Part model, mm, in its own coordinate system. A direction names the side the tool comes from. Give positions to 0.01 mm unless a question says otherwise; leave off trailing zeros. Write each loop counter-clockwise with the first axis right and the second up, starting at its lowest first coordinate (ties: lowest second). Pieces come first, ordered by that corner, then holes. Notation, with made-up numbers: (56, 84) - (110, 84) arc R12 ccw to (110, 105) - close; hole circle Ø2 at (18.25, 50). An arc over 180 degrees is marked (long way). Answer in a Markdown table with one row per item. Add a question column.
1. Pull direction Y, two halves, no side cores. Call faces 5 (the cylindrical face through (3.22, 1.01, 3.03)), 6 (the conical face through (1.35, 3.27, 5.16)), 7 (the flat face through (6.7, -0.1, 1.2)), 8 (the flat face through (0, 8, 3)): released by +Y, released by -Y, zero draft, split by the parting line, or undercut.
2. Band-saw the part on D-D on x = -7. Write the cut outline in (y, z).
3. Band-saw the part on B-B on z = 3. Write the cut outline in (x, y) (3 decimals), plus the area to 3 significant figures.
4. Band-saw the part on A-A on y = 0. Write the cut outline in (x, z) (3 decimals).
5. Probe line 1 along X through (y, z) = (0, 3.55) (3 decimals); line 2 along Y through (x, z) = (-1.5, 1.5). List the from-to ranges inside material, lowest first.
6. Drop flat-ended pins along their axis: pin 1 Ø1.7 at (x, y) = (-6, 2) entering from +Z; pin 2 Ø1.4 at (y, z) = (-0.5, 5) entering from -X; pin 3 Ø1 at (y, z) = (3, 5.5) entering from +X. Give the stop position or say it passes through.
7. Band-saw the part on C-C on y = 5.25. Write the cut outline in (x, z), plus the area to 3 significant figures.
8. Which spindle directions (+Z, -Z, +X, -X, +Y, -Y) get a long thin tool onto all of the face, cutting with end or side? Do faces 1 (the flat face through (4, 0, 5)), 2 (the flat face through (-6.8, -0.1, 1.3)), 3 (the flat face through (-6, 0, 4.1)), 4 (the flat face through (-0.493, 5.868, 5.706)). Say none if no direction does.
```python
from build123d import *

# Parameters (mm, degrees)
PAD_DEPTH   = 8
SKETCH001_R = 3.375
HOLE_DEPTH  = 6.001


with BuildPart() as part:
    # Sketch → Pad (new body, symmetric)
    with BuildSketch(Plane.XZ):
        with BuildLine():
            Line((-1, 6), (-3.7, 6))
            ThreePointArc((-3.7, 6), (-3.912132, 5.912132), (-4, 5.7))
            Line((-4, 5.7), (-4, 4.4))
            ThreePointArc((-4.3, 4.1), (-4.087868, 4.187868), (-4, 4.4))
            Line((-4.3, 4.1), (-7.7, 4.1))
            ThreePointArc((-7.7, 4.1), (-7.912132, 4.012132), (-8, 3.8))
            Line((-8, 3.8), (-8, 2.624264))
            ThreePointArc((-8, 2.624264), (-7.977164, 2.509459), (-7.912132, 2.412132))
            Line((-7.912132, 2.412132), (-5.587868, 0.087868))
            ThreePointArc((-5.587868, 0.087868), (-5.490541, 0.022836), (-5.375736, 0))
            Line((-5.375736, 0), (5.375736, 0))
            ThreePointArc((5.375736, 0), (5.490541, 0.022836), (5.587868, 0.087868))
            Line((5.587868, 0.087868), (7.912132, 2.412132))
            ThreePointArc((7.912132, 2.412132), (7.977164, 2.509459), (8, 2.624264))
            Line((8, 2.624264), (8, 3.8))
            ThreePointArc((8, 3.8), (7.912132, 4.012132), (7.7, 4.1))
            Line((7.7, 4.1), (4.3, 4.1))
            ThreePointArc((4, 4.4), (4.087868, 4.187868), (4.3, 4.1))
            Line((4, 4.4), (4, 5.7))
            ThreePointArc((4, 5.7), (3.912132, 5.912132), (3.7, 6))
            Line((3.7, 6), (1, 6))
            Line((1, 6), (0, 5.42))
            Line((0, 5.42), (-1, 6))
        make_face()
    extrude(amount=PAD_DEPTH, both=True)

    # Sketch001 → Hole (cut, through all)
    with BuildSketch(Plane.XY.offset(6)):
        Circle(SKETCH001_R)
    extrude(amount=-HOLE_DEPTH, mode=Mode.SUBTRACT)

    # Sketch002 → Groove (revolve, cut)
    with BuildSketch(Plane.YZ):
        Polygon((3.375, 6), (4.375, 6), (3.375, 5), align=None)
        Polygon((3.375, 0), (3.375, 1), (4.375, 0), align=None)
    revolve(axis=Axis((0, 0, 0), (0, 0, 1)), mode=Mode.SUBTRACT)


solid = part.part
```
Values:
| question | item | result |
|---|---|---|
| 1 | face 5 | undercut |
| 1 | face 6 | undercut |
| 1 | face 7 | zero draft |
| 1 | face 8 | released by +Y |
| 2 | outline | (-8, 1.5) - (8, 1.5) - (8, 4.1) - (-8, 4.1) - close |
| 3 | outline | (-8, -8) - (8, -8) - (8, 8) - (-8, 8) - close; hole circle Ø6.75 at (0, 0) |
| 3 | area | 220 mm² |
| 4 | outline | (-8, 2.624) arc R0.3 ccw to (-7.912, 2.412) - (-5.588, 0.088) arc R0.3 ccw to (-5.376, 0) - (-4.375, 0) - (-3.375, 1) - (-3.375, 5) - (-4, 5.625) - (-4, 4.4) arc R0.3 cw to (-4.3, 4.1) - (-7.7, 4.1) arc R0.3 ccw to (-8, 3.8) - close; (3.375, 1) - (4.375, 0) - (5.376, 0) arc R0.3 ccw to (5.588, 0.088) - (7.912, 2.412) arc R0.3 ccw to (8, 2.624) - (8, 3.8) arc R0.3 ccw to (7.7, 4.1) - (4.3, 4.1) arc R0.3 cw to (4, 4.4) - (4, 5.625) - (3.375, 5) - close |
| 5 | line 1 | x = -8 to -3.375, 3.375 to 8 |
| 5 | line 2 | y = -8 to -3.02, 3.02 to 8 |
| 6 | pin 1 | stops at z = 4.1 |
| 6 | pin 2 | stops at x = -4.02 |
| 6 | pin 3 | stops at x = 4 |
| 7 | outline | (-8, 2.62) arc R0.3 ccw to (-7.91, 2.41) - (-5.59, 0.09) arc R0.3 ccw to (-5.38, 0) - (5.38, 0) arc R0.3 ccw to (5.59, 0.09) - (7.91, 2.41) arc R0.3 ccw to (8, 2.62) - (8, 3.8) arc R0.3 ccw to (7.7, 4.1) - (4.3, 4.1) arc R0.3 cw to (4, 4.4) - (4, 5.7) arc R0.3 ccw to (3.7, 6) - (1, 6) - (0, 5.42) - (-1, 6) - (-3.7, 6) arc R0.3 ccw to (-4, 5.7) - (-4, 4.4) arc R0.3 cw to (-4.3, 4.1) - (-7.7, 4.1) arc R0.3 ccw to (-8, 3.8) - close |
| 7 | area | 73.9 mm² |
| 8 | face 1 | +Z, +X, +Y, -Y |
| 8 | face 2 | -Z, -X, +Y, -Y |
| 8 | face 3 | +Z, -X, +Y, -Y |
| 8 | face 4 | +Z, +Y, -Y |
